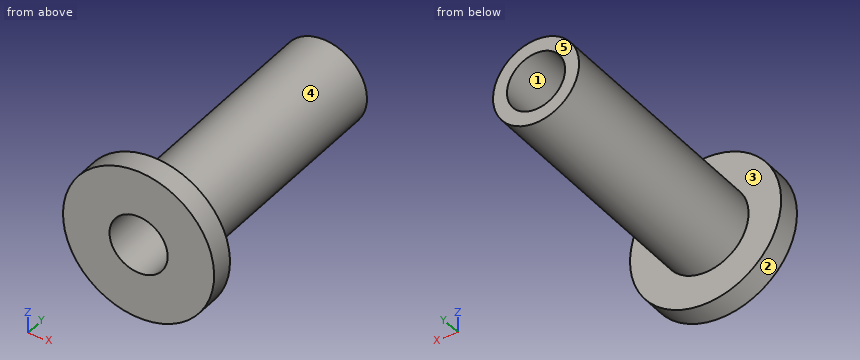
from build123d import *

# Parameters (mm, degrees)
SKETCH1_R           = 4.1275
BOSS_EXTRUDE1_DEPTH = 1.27
SKETCH2_R           = 2.3495
BOSS_EXTRUDE2_DEPTH = 13.589
SKETCH3_R           = 1.5875
CUT_EXTRUDE2_DEPTH  = 16.964410215


with BuildPart() as part:
    # Sketch1 → Boss-Extrude1 (new body)
    with BuildSketch(Plane(origin=(0, 0, 0), x_dir=(1, 0, 0), z_dir=(0, 1, 0))):
        with Locations(Location((0, 0, 0), (0, 0, 270))):
            Circle(SKETCH1_R)
    extrude(amount=BOSS_EXTRUDE1_DEPTH)

    # Sketch2 → Boss-Extrude2 (add)
    with BuildSketch(Plane(origin=(0, 1.27, 0), x_dir=(1, 0, 0), z_dir=(0, 1, 0))):
        with Locations(Location((0, 0, 0), (0, 0, 270))):
            Circle(SKETCH2_R)
    extrude(amount=BOSS_EXTRUDE2_DEPTH)

    # Sketch3 → Cut-Extrude2 (cut, through all)
    with BuildSketch(Plane.XZ):
        with Locations(Location((0, 0, 0), (0, 0, 270))):
            Circle(SKETCH3_R)
    extrude(amount=-CUT_EXTRUDE2_DEPTH, mode=Mode.SUBTRACT)


solid = part.part
Here's how the part is built. I have some questions about the finished solid (model axes, mm). Face numbers are marked on the shaded views. A direction names the side the tool comes from. Round coordinates to 2 decimals unless told otherwise and drop trailing zeros. Write each loop counter-clockwise with the first axis right and the second up, starting at its lowest first coordinate (ties: lowest second). Pieces come first, ordered by that corner, then holes.
1. I need wall thicknesses on L1, parallel to X at y = 8, z = 0; L2, parallel to Y at x = 2.5, z = 0.5; L3, parallel to Z at x = -0.25, y = 5.5. Which ranges of each line are inside material? Lowest first, please.
2. Suppose I cut it at D-D (z = -2). List the corners of the cut face in (x, y) for me, and give its area (3 significant figures).
3. Suppose I cut it at A-A (x = 0). List the corners of the cut face in (y, z) for me.
4. Suppose I cut it at C-C (y = 8.75). List the corners of the cut face in (x, z) for me (1 decimal).
5. For the marked faces 4 and 5, which set-ups out of +Z, -Z, +X, -X, +Y, -Y let a thin tool reach every point of the face, with its end or its side?
6. Suppose I cut it at B-B (z = 0). List the corners of the cut face in (x, y) for me, and give its area (3 significant figures).
7. Will these pins go through, and if not, where does the flat tip stop? pin 1 Ø1 at (y, z) = (9.5, 0.5) entering from +X; pin 2 Ø3 at (y, z) = (2, -2) entering from +X; pin 3 Ø2 at (x, y) = (-2.5, 10.5) entering from +Z.
8. If we mould it in two halves opening along Z, with no side actions, what happens to the marked faces 1, 2 and 3? For each: released by +Z, released by -Z, zero draft, split by the parting line, or undercut.
Answer sheet:
1. L1: x = -2.35 to -1.59, 1.59 to 2.35
1. L2: y = 0 to 1.27
1. L3: z = -2.34 to -1.57, 1.57 to 2.34
2. outline: (-3.61, 0) - (3.61, 0) - (3.61, 1.27) - (1.23, 1.27) - (1.23, 14.86) - (-1.23, 14.86) - (-1.23, 1.27) - (-3.61, 1.27) - close
2. area: 42.7 mm2
3. outline: (0, -4.13) - (1.27, -4.13) - (1.27, -2.35) - (14.86, -2.35) - (14.86, -1.59) - (0, -1.59) - close; (0, 1.59) - (14.86, 1.59) - (14.86, 2.35) - (1.27, 2.35) - (1.27, 4.13) - (0, 4.13) - close
4. outline: circle Ø4.7 at (0, 0); hole circle Ø3.2 at (0, 0)
5. face 4: +Y
5. face 5: +Z, -Z, +X, -X, +Y
6. outline: (-4.13, 0) - (-1.59, 0) - (-1.59, 14.86) - (-2.35, 14.86) - (-2.35, 1.27) - (-4.13, 1.27) - close; (1.59, 0) - (4.13, 0) - (4.13, 1.27) - (2.35, 1.27) - (2.35, 14.86) - (1.59, 14.86) - close
6. area: 27.2 mm2
7. pin 1: stops at x = 2.35
7. pin 2: stops at x = 4.07
7. pin 3: stops at z = 1.81
8. face 1: undercut
8. face 2: split by the parting line
8. face 3: zero draft
